```python
from build123d import *

# Parameters (mm, degrees)
SKETCH1_W           = 150
SKETCH1_H           = 85
BOSS_EXTRUDE1_DEPTH = 3
SKETCH2_R           = 2
CUT_EXTRUDE1_DEPTH  = 3
SKETCH3_R           = 2
CUT_EXTRUDE2_DEPTH  = 3
CUT_EXTRUDE4_REACH  = 5
SKETCH5_W           = 19
SKETCH5_H           = 12


with BuildPart() as part:
    # Sketch1 → Boss-Extrude1 (new body)
    with BuildSketch(Plane.XY):
        Rectangle(SKETCH1_W, SKETCH1_H)
    extrude(amount=BOSS_EXTRUDE1_DEPTH)

    # Sketch2 → Cut-Extrude1 (cut)
    with BuildSketch(Plane.XY.offset(3)):
        with Locations((-30, 26.5)):
            Circle(SKETCH2_R)
    cut_extrude1 = extrude(amount=-CUT_EXTRUDE1_DEPTH, mode=Mode.SUBTRACT)

    # Mirror1: Cut-Extrude1 across plane
    add(cut_extrude1.mirror(Plane(origin=(0, 0, 0), x_dir=(0, 0, 1), z_dir=(1, 0, 0))), mode=Mode.SUBTRACT)

    # Sketch3 → Cut-Extrude2 (cut)
    with BuildSketch(Plane.XY.offset(3)):
        with Locations((-59, 0)):
            Circle(SKETCH3_R)
    cut_extrude2 = extrude(amount=-CUT_EXTRUDE2_DEPTH, mode=Mode.SUBTRACT)

    # Mirror2: Cut-Extrude2 across plane
    add(cut_extrude2.mirror(Plane(origin=(0, 0, 0), x_dir=(0, 0, 1), z_dir=(1, 0, 0))), mode=Mode.SUBTRACT)

    # Sketch5 → Cut-Extrude4 (cut, up to next)
    with BuildSketch(Plane.XY.offset(3), mode=Mode.PRIVATE) as cut_extrude4_sk1:
        with Locations((-30, 16.5)):
            Rectangle(SKETCH5_W, SKETCH5_H)
    cut_extrude4_tool1 = extrude(cut_extrude4_sk1.sketch, amount=-CUT_EXTRUDE4_REACH, mode=Mode.PRIVATE) & part.part
    add(cut_extrude4_tool1.solids().sort_by_distance((-30, 16.5, 3))[0], mode=Mode.SUBTRACT)


solid = part.part
```
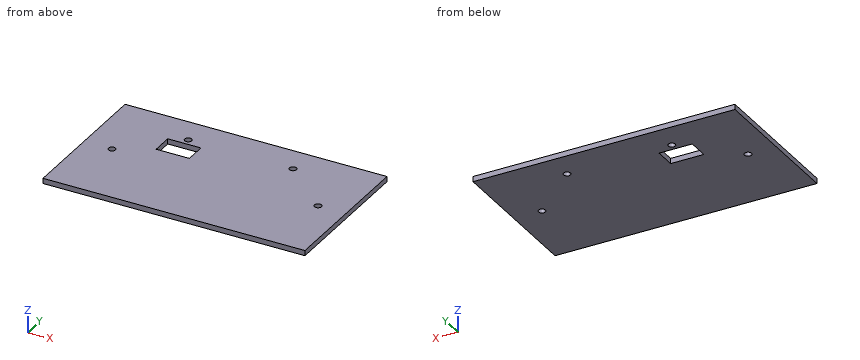
Could you check a few things on this model? Use its own coordinates, in mm. Round coordinates to 2 decimals unless told otherwise and drop trailing zeros. Order: outer loops, then holes, each group sorted by start corner. A loop starts at its lowest first (then second) coordinate and runs counter-clockwise, first axis right, second up. Notation, with made-up numbers: M 40,70 L 51,70 A22 cw 51,83 Z; hole C 35.5,-32 d5. An arc over 180 degrees is marked long. One line per question, with ' | ' between items. Start each with the question number.
(1) Suppose I cut it at B-B on x = 30. List the corners of the cut face in (y, z) for me.
(2) For P1, Ø2.5, axis at x = -30, y = 26.5, coming from the +Z side, with a flat end and sliding along its axis, tell me the tip position at first contact or that it passes through.
(3) Please list where these lines run through material, in increasing order: line 1 along Y through (x, z) = (-30, 1.75); line 2 along Y through (x, z) = (-59, 2.2); line 3 along Y through (x, z) = (-36, 2.3).
(4) Suppose I cut it at A-A on y = 20.5. List the corners of the cut face in (x, z) for me.
(5) Suppose I cut it at C-C on z = 0.5. List the corners of the cut face in (x, y) for me, then the cut area to 3 significant figures.
(6) Suppose I cut it at D-D on y = 0. List the corners of the cut face in (x, z) for me, then the cut area to 3 significant figures.
Geometry results:
1) outline: M -42.5,0 L 24.5,0 L 24.5,3 L -42.5,3 Z; M 28.5,0 L 42.5,0 L 42.5,3 L 28.5,3 Z
2) P1: through
3) line 1: -42.5 to 10.5, 22.5 to 24.5, 28.5 to 42.5 | line 2: -42.5 to -2, 2 to 42.5 | line 3: -42.5 to 10.5, 22.5 to 42.5
4) outline: M -75,0 L -39.5,0 L -39.5,3 L -75,3 Z; M -20.5,0 L 75,0 L 75,3 L -20.5,3 Z
5) outline: M -75,-42.5 L 75,-42.5 L 75,42.5 L -75,42.5 Z; hole C -59,0 d4; hole M -39.5,10.5 L -20.5,10.5 L -20.5,22.5 L -39.5,22.5 Z; hole C -30,26.5 d4; hole C 30,26.5 d4; hole C 59,0 d4 | area: 12,500 mm²
6) outline: M -75,0 L -61,0 L -61,3 L -75,3 Z; M -57,0 L 57,0 L 57,3 L -57,3 Z; M 61,0 L 75,0 L 75,3 L 61,3 Z | area: 426 mm²
